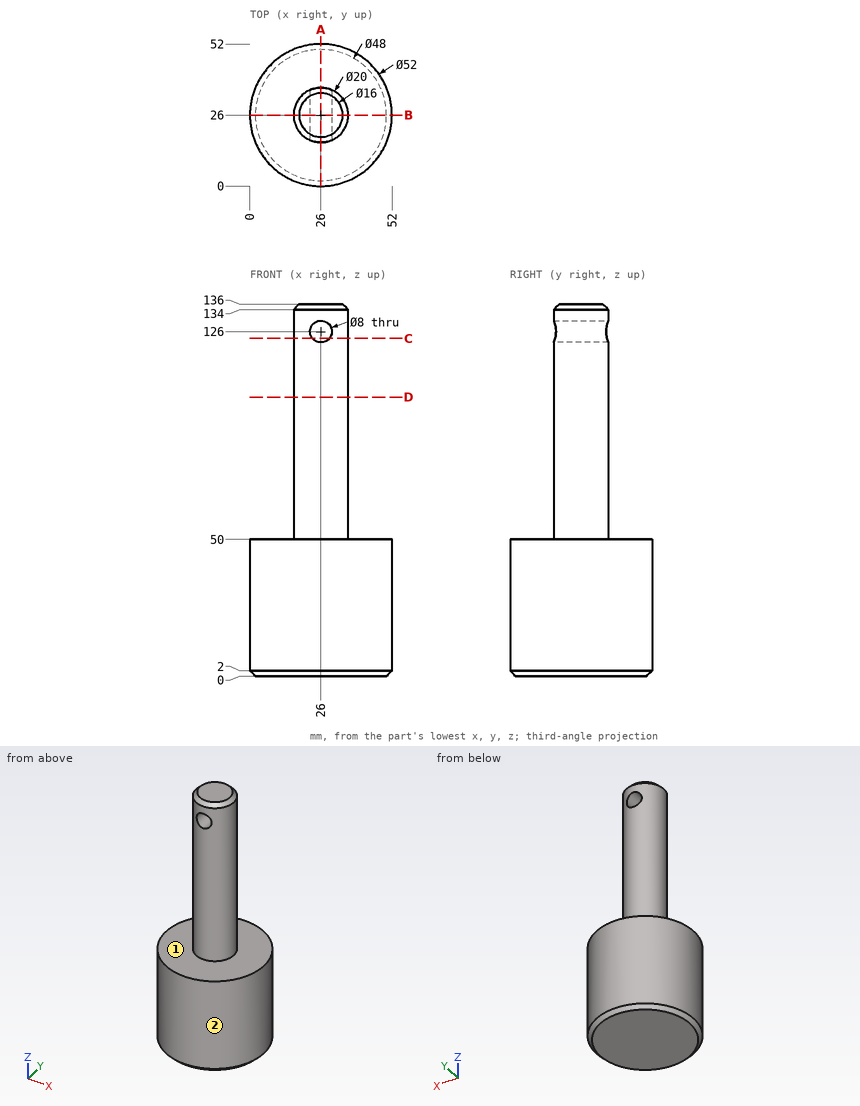
Here's the drawing with two shaded views (mm, measured from the low corner). I have some questions. A direction names the side the tool comes from. Round coordinates to 2 decimals unless told otherwise and drop trailing zeros. Loops run counter-clockwise (first coordinate to the right, second up) from the corner with the lowest first, then second, coordinate; pieces in that order, holes last.
Item 1: Suppose I cut it at B-B, the plane y = 26. Write out the boundary of the cut face in (x, z).
Item 2: Please list where these lines run through material, in increasing order: L1, parallel to Z at x = 26, y = 29; L2, parallel to X at y = 22, z = 126; L3, parallel to Z at x = 36, y = 18.
Item 3: Suppose I cut it at A-A, the plane x = 26. Write out the boundary of the cut face in (y, z).
Item 4: Suppose I cut it at C-C, the plane z = 123.5. Write out the boundary of the cut face in (x, y), then the cut area to 3 significant figures.
Item 5: Suppose I cut it at D-D, the plane z = 102. Write out the boundary of the cut face in (x, y), then the cut area to 3 significant figures.
Item 6: Which directions (+Z, -Z, +X, -X, +Y, -Y) give clear straight access to the entire face, cutting with the end or side of a thin tool? Please do the marked faces 1 and 2.
Item 7: Will these pins go through, and if not, where does the flat tip stop? pin 1 Ø8 at (x, z) = (38, 97) entering from -Y; pin 2 Ø6.5 at (x, z) = (26, 126) entering from -Y; pin 3 Ø5 at (x, z) = (27.5, 63.5) entering from +Y; pin 4 Ø4 at (x, z) = (23.5, 117) entering from -Y.
Reported:
1. outline: (0, 2) - (2, 0) - (50, 0) - (52, 2) - (52, 50) - (36, 50) - (36, 134) - (34, 136) - (18, 136) - (16, 134) - (16, 50) - (0, 50) - close; hole circle Ø8 at (26, 126)
2. L1: z = 0 to 122, 130 to 136
2. L2: x = 16.83 to 22, 30 to 35.17
2. L3: z = 0 to 50
3. outline: (0, 2) - (2, 0) - (50, 0) - (52, 2) - (52, 50) - (36, 50) - (36, 122) - (16, 122) - (16, 50) - (0, 50) - close; (16, 130) - (36, 130) - (36, 134) - (34, 136) - (18, 136) - (16, 134) - close
4. outline: (22.88, 16.5) - (22.88, 35.5) arc R10 ccw to start; (29.12, 16.5) arc R10 ccw to (29.12, 35.5) - close
4. area: 191 mm2
5. outline: circle Ø20 at (26, 26)
5. area: 314 mm2
6. face 1: +Z
6. face 2: +Z, -Z
7. pin 1: stops at y = 20
7. pin 2: passes through
7. pin 3: stops at y = 36
7. pin 4: stops at y = 16.01
